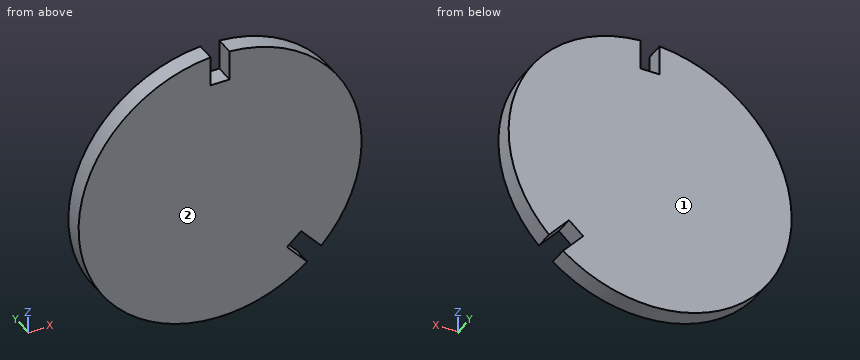
```python
from build123d import *

# Parameters (mm, degrees)
F1_DEPTH = 0.635


with BuildPart() as f1:
    # F0 (on Front) → F1 (new body, symmetric)
    with BuildSketch(Plane.XZ):
        with BuildLine():
            Line((5.454479, -5.145855), (6.809138, -6.660426))
            ThreePointArc((6.809138, -6.660426), (8.898001, 3.398706), (0.635, 9.50381))
            Line((0.635, 9.50381), (0.635, 7.47181))
            Line((0.635, 7.47181), (-0.635, 7.47181))
            Line((-0.635, 7.47181), (-0.635, 9.50381))
            ThreePointArc((-0.635, 9.50381), (-8.898001, -3.398706), (5.862531, -7.507087))
            Line((5.862531, -7.507087), (4.507873, -5.992516))
            Line((4.507873, -5.992516), (5.454479, -5.145855))
        make_face()
    extrude(amount=F1_DEPTH, both=True)


solid = f1.part
```
Verification items for the finished model (mm, model axes). Face numbers are marked on the shaded views. Coordinates: 2 decimals unless noted, no trailing zeros. Loops run counter-clockwise (first coordinate to the right, second up) from the corner with the lowest first, then second, coordinate; pieces in that order, holes last. Notation, with made-up numbers: (80.5, 21) - (122.5, 21) arc R23 cw to (122.5, 44) - close; hole circle Ø6 at (-38.75, 41). An arc over 180 degrees is marked (long way). Return JSON: item names as keys, results as strings.
1. Thickness scan on L1, parallel to Z at x = -8.25, y = 0.2; L2, parallel to X at y = -0.45, z = 0.25. Record the ranges inside material, lowest first.
Established:
{"L1": "z = -4.76 to 4.76", "L2": "x = -9.52 to 9.52"}
2. Section check A-A, the plane y = -0.15. Record the boundary of the cut face in (x, z) (3 decimals).
Established:
{"outline": "(-0.635, 7.472) - (-0.635, 9.504) arc R9.525 ccw (long way) to (5.863, -7.507) - (4.508, -5.993) - (5.454, -5.146) - (6.809, -6.66) arc R9.525 ccw to (0.635, 9.504) - (0.635, 7.472) - close"}
3. Section check B-B, the plane x = 0. Record the boundary of the cut face in (y, z) (3 decimals).
Established:
{"outline": "(-0.635, -9.525) - (0.635, -9.525) - (0.635, 7.472) - (-0.635, 7.472) - close"}
4. Mould release check, pull along Y, two halves, no side actions. Record for the marked faces 1 and 2: +Y half, -Y half, draft (parallel to the pull), parting line (faces both ways), or undercut.
Established:
{"face 1": "+Y half", "face 2": "-Y half"}
5. Go/stop test with flat-tipped pins: pin 1 (0.6 mm diameter, centred on y = 0, z = 8.5, fed in from -X); pin 2 (0.6 mm diameter, centred on x = 0, y = 0.5, fed in from +Z); pin 3 (0.6 mm diameter, centred on y = 0, z = 8.5, fed in from +X). Record where each tip stops, or that it passes through.
Established:
{"pin 1": "stops at x = -4.85", "pin 2": "stops at z = 7.47", "pin 3": "stops at x = 4.85"}
6. Section check C-C, the plane z = 6.25. Record the boundary of the cut face in (x, y) (3 decimals).
Established:
{"outline": "(-7.188, -0.635) - (7.188, -0.635) - (7.188, 0.635) - (-7.188, 0.635) - close"}
